Can you work these out from the model? Positions are in its coordinate system, mm. Give positions to 0.01 mm unless a question says otherwise; leave off trailing zeros. Order: outer loops, then holes, each group sorted by start corner. A loop starts at its lowest first (then second) coordinate and runs counter-clockwise, first axis right, second up. Notation, with made-up numbers: M 69.5,88.5 L 101.5,88.5 A31 ccw 101.5,120.5 Z; hole C -38.75,30.5 d10. An arc over 180 degrees is marked long. Answer as a JSON object with one key per item and string values.
```python
from build123d import *

# Parameters (mm, degrees)
SKETCH1_W            = 30
SKETCH1_H            = 10
BOSS_EXTRUDE1_DEPTH  = 3
M3_CLEARANCE_HOLE1_D = 3.4
FILLET3_R            = 1
CUT_EXTRUDE4_START   = -10
CUT_EXTRUDE4_DEPTH   = 10
FILLET4_R            = 0.5


# Read off the part's stored shape, not the designer's step: Cut-Extrude4
with BuildPart() as part:
    # Sketch1 → Boss-Extrude1 (new body)
    with BuildSketch(Plane(origin=(0, 0, 0), x_dir=(1, 0, 0), z_dir=(0, 1, 0))):
        with Locations((8.769230769, -2)):
            Rectangle(SKETCH1_W, SKETCH1_H)
    extrude(amount=BOSS_EXTRUDE1_DEPTH)

    # M3 Clearance Hole1 (through all)
    with Locations(Plane(origin=(0, 3, 0), x_dir=(1, 0, 0), z_dir=(0, 1, 0))):
        with Locations((-2.230769231, -2), (19.269230769, -2)):
            Hole(M3_CLEARANCE_HOLE1_D / 2)

    # Fillet3
    fillet3_edges = [part.edges().sort_by_distance(p)[0] for p in [
        (8.769230769, 3, 7),
        (23.769230769, 3, 2),
        (8.769230769, 3, -3),
        (-6.230769231, 3, 2),
    ]]
    fillet(fillet3_edges, radius=FILLET3_R)

    # Cut-Extrude4 outline → Cut-Extrude4 (cut)
    with BuildSketch(Plane.XY.offset(7).offset(CUT_EXTRUDE4_START)):
        with BuildLine():
            ThreePointArc((23.769230769, 0), (8.769230769, 0.426355955), (-6.230769231, 0))
            Line((-6.230769231, 0), (23.769230769, 0))
        make_face()
    extrude(amount=CUT_EXTRUDE4_DEPTH, mode=Mode.SUBTRACT)

    # Fillet4
    fillet4_edges = [part.edges().sort_by_distance(p)[0] for p in [
        (23.769230769, 0, 2),
        (-6.230769231, 0, 2),
    ]]
    fillet(fillet4_edges, radius=FILLET4_R)


solid = part.part
```
1) I need wall thicknesses on L1, parallel to X at y = 0.8, z = 1.25; L2, parallel to Y at x = 8.5, z = -0.5; L3, parallel to X at y = 1.5, z = 0.5. Which ranges of each line are inside material? Lowest first, please.
Results found:
{"L1": "x = -6.23 to -3.76, -0.71 to 17.74, 20.79 to 23.77", "L2": "y = 0.43 to 3", "L3": "x = -6.23 to -3.03, -1.43 to 18.47, 20.07 to 23.77"}
2) I want a section at D-D on x = 6.5. Write out the boundary of the cut face in (y, z).
Results found:
{"outline": "M 0.42,-3 L 2,-3 A1 ccw 3,-2 L 3,6 A1 ccw 2,7 L 0.42,7 Z"}
3) I want a section at A-A on x = -1.5. Write out the boundary of the cut face in (y, z).
Results found:
{"outline": "M 0.23,-3 L 2,-3 A1 ccw 3,-2 L 3,0.47 L 0.23,0.47 Z; M 0.23,3.53 L 3,3.53 L 3,6 A1 ccw 2,7 L 0.23,7 Z"}
4) I'm going to push flat-ended pins straight in: pin 1 Ø2 at (x, z) = (19, 0.5) entering from -Y; pin 2 Ø2 at (x, z) = (-2.23, 2) entering from +Y. Where does each tip first touch, or does it pass through?
Results found:
{"pin 1": "stops at y = 0.19", "pin 2": "passes through"}
5) Thinking about a two-plate mould opening in Z: for faces 1 (the face through (8.979, 2.699, -2.715)), 2 (the face through (-3.852, 1.54, 1.489)), 3 (the face through (23.769, 1, 2)), which applies, pulls with the +Z half, pulls with the -Z half, needs draft (parallel to the pull), parting line crosses it, or undercut?
Results found:
{"face 1": "pulls with the -Z half", "face 2": "undercut", "face 3": "needs draft"}
6) I want a section at B-B on z = 1. Write out the boundary of the cut face in (x, y).
Results found:
{"outline": "M -6.23,0.53 A0.5 ccw -5.7,0.03 A264.08 cw -3.61,0.14 L -3.61,3 L -5.23,3 A1 ccw -6.23,2 Z; M -0.86,0.25 A264.08 cw 17.89,0.27 L 17.89,3 L -0.86,3 Z; M 20.64,0.16 A264.08 cw 23.24,0.03 A0.5 ccw 23.77,0.53 L 23.77,2 A1 ccw 22.77,3 L 20.64,3 Z"}
7) I want a section at C-C on y = 1.45. Write out the boundary of the cut face in (x, z).
Results found:
{"outline": "M -6.23,-3 L 23.77,-3 L 23.77,7 L -6.23,7 Z; hole C -2.23,2 d3.4; hole C 19.27,2 d3.4"}
